Autodesk Inventor part; units mm, degrees
ref_plane "YZ Plane" through (0, 0, 0) normal (1, 0, 0) x (0, 1, 0)
ref_plane "XZ Plane" through (0, 0, 0) normal (0, 1, 0) x (-1, 0, 0)
ref_plane "XY Plane" through (0, 0, 0) normal (0, 0, 1) x (1, 0, 0)
sketch "Sketch1" plane through (0, 0, 0) normal (0, 0, 1) x (1, 0, 0)
  circle A0 centre (0, 0) radius 4
  arc A1 (7.5, 0) -> (-7.5, 0) centre (0, 0) ccw
  line L0 (-7.5, 0) -> (7.5, 0)
  line L1 (7.5, 0) -> (7.5, -30)
  line L2 (7.5, -30) -> (-7.5, -30)
  line L3 (-7.5, -30) -> (-7.5, 0)
  dimension "d0" = 8
  dimension "d1" = 15
  dimension "d2" = 15
  dimension "d3" = 30
extrude "Extrusion1" add sketch "Sketch1" along normal mid plane 5 contours L0 L1 L2 L3 A0 | A0 L0 A1
sketch "Sketch2" plane through (0, 0, -2.5) normal (0, 0, -1) x (-1, 0, 0)
  line L0 (7.5, -30) -> (-7.5, -30)
  line L1 (-7.5, -30) -> (7.5, -30)
  line L2 (7.5, -30) -> (7.5, -27.5)
  line L3 (7.5, -27.5) -> (-7.5, -27.5)
  line L4 (-7.5, -27.5) -> (-7.5, -30)
  point P0 (0, 0)
  point P1 (7.5, -30)
  dimension "d6" = 15
  dimension "d7" = 2.5
extrude "Extrusion2" add sketch "Sketch2" along normal blind 44
sketch "Sketch3" plane through (-7.5, -27.5, -2.5) normal (0, 1, 0) x (1, 0, 0)
  line L0 (0, -5) -> (15, -5)
  line L1 (7.5, -5) -> (7.5, 4.5)
  line L2 (7.5, 4.5) -> (7.5, 34.5)
  point P0 (7.5, -2.5)
  dimension "d10" = 9.5
  dimension "d11" = 30
hole "Hole1" at (0, -27.5, -7) at (0, -27.5, -37) direction (0, -1, 0) diameter 4 depth 6
properties part number "Half Bearing Block"
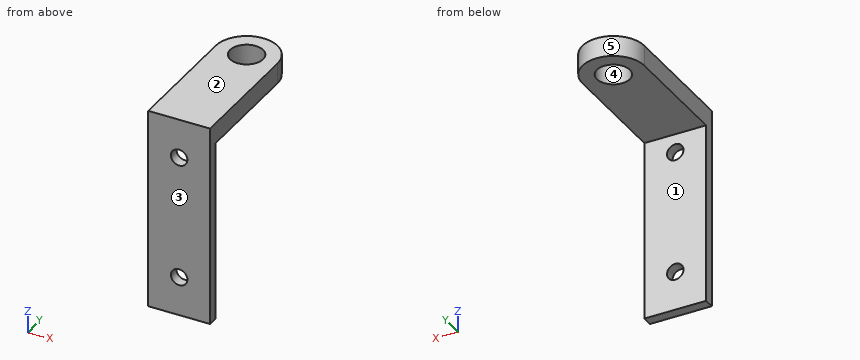
Verification items for the finished model (mm, model axes). Face numbers are marked on the shaded views. A direction names the side the tool comes from. Give positions to 0.01 mm unless a question says otherwise; leave off trailing zeros. Order: outer loops, then holes, each group sorted by start corner. A loop starts at its lowest first (then second) coordinate and runs counter-clockwise, first axis right, second up. Notation, with made-up numbers: (-6, 13) - (28, 13) arc R11 ccw to (28, 19) - close; hole circle Ø9 at (-39, -19). An arc over 180 degrees is marked (long way). Answer as CSV lines item,"result". Start each with the question number.
Item 1: Mould release check, pull along Y, two halves, no side actions. Record for the marked faces 3, 4 and 5: released by +Y, released by -Y, zero draft, split by the parting line, or undercut.
Item 2: Access from +Z, -Z, +X, -X, +Y, -Y to the whole of each face (thin tool, end or side, straight path). Record for the marked faces 1 and 2.
Item 3: Gauge pin test, flat ends, axial feed: pin 1 (5 mm diameter, centred on x = 0, y = 0, fed in from +Z); pin 2 (7.5 mm diameter, centred on x = 2, z = -15.5, fed in from +Y); pin 3 (4.5 mm diameter, centred on x = 1, y = -7, fed in from -Z). Record the tip position at first contact, or that the pin passes through.
Item 4: Section check B-B, the plane x = 0. Record the boundary of the cut face in (y, z), plus the area to 4 significant figures.
Item 5: Material ranges on L1, parallel to Z at x = 0, y = -28.75; L2, parallel to X at y = -29, z = -7; L3, parallel to Y at x = -5.75, z = -11, recorded low to high.
Item 6: Section check C-C, the plane y = -2.5. Record the boundary of the cut face in (x, z).
Item 7: Section check A-A, the plane z = -7. Record the boundary of the cut face in (x, y), plus the area to 3 significant figures.
Item 8: Section check D-D, the plane x = -6. Record the boundary of the cut face in (y, z).
Filled in:
1,face 3,"released by -Y"
1,face 4,"undercut"
1,face 5,"released by +Y"
2,face 1,"-Z, +X, -X, +Y"
2,face 2,"+Z, +X, -X, +Y, -Y"
3,pin 1,"through"
3,pin 2,"y = -27.5"
3,pin 3,"z = -2.5"
4,outline,"(-30, -46.5) - (-27.5, -46.5) - (-27.5, -39) - (-30, -39) - close; (-30, -35) - (-27.5, -35) - (-27.5, -9) - (-30, -9) - close; (-30, -5) - (-27.5, -5) - (-27.5, -2.5) - (-4, -2.5) - (-4, 2.5) - (-30, 2.5) - close; (4, -2.5) - (7.5, -2.5) - (7.5, 2.5) - (4, 2.5) - close"
4,area,"237.5 mm^2"
5,L1,"-46.5 to -39, -35 to -9, -5 to 2.5"
5,L2,"-7.5 to -2, 2 to 7.5"
5,L3,"-30 to -27.5"
6,outline,"(-7.5, -2.5) - (-3.12, -2.5) - (-3.12, 2.5) - (-7.5, 2.5) - close; (3.12, -2.5) - (7.5, -2.5) - (7.5, 2.5) - (3.12, 2.5) - close"
7,outline,"(-7.5, -30) - (-2, -30) - (-2, -27.5) - (-7.5, -27.5) - close; (2, -30) - (7.5, -30) - (7.5, -27.5) - (2, -27.5) - close"
7,area,"27.5 mm^2"
8,outline,"(-30, -46.5) - (-27.5, -46.5) - (-27.5, -2.5) - (4.5, -2.5) - (4.5, 2.5) - (-30, 2.5) - close"
